Geometry check sheet. Reference: the model listing, model coordinates, mm. A direction names the side the tool comes from. Coordinates: 2 decimals unless noted, no trailing zeros. Loops run counter-clockwise (first coordinate to the right, second up) from the corner with the lowest first, then second, coordinate; pieces in that order, holes last. Notation, with made-up numbers: (-12.75, 11.25) -> (9.25, 11.25) arc R29 cw to (9.25, 31.25) -> close; hole circle Ø3 at (-25.5, -12.5). An arc over 180 degrees is marked (long way). Answer as a JSON object with one key per item and string values.
from build123d import *

# Parameters (mm, degrees)
SKETCH1_R           = 2.8
BOSS_EXTRUDE1_DEPTH = 1.5
SKETCH2_R           = 2.25
BOSS_EXTRUDE2_DEPTH = 7
SKETCH3_R           = 2.25
BOSS_EXTRUDE3_DEPTH = 15
CUT_EXTRUDE1_DEPTH  = 103.8
SKETCH5_R           = 1.8
CUT_EXTRUDE2_DEPTH  = 116.0000001
CUT_EXTRUDE3_DEPTH  = 13.8


with BuildPart() as part:
    # Sketch1 → Boss-Extrude1 (new body)
    with BuildSketch(Plane(origin=(0, 0, 0), x_dir=(1, 0, 0), z_dir=(0, 1, 0))):
        Circle(SKETCH1_R)
    extrude(amount=BOSS_EXTRUDE1_DEPTH)

    # Sketch2 → Boss-Extrude2 (add)
    with BuildSketch(Plane(origin=(0, 1.5, 0), x_dir=(1, 0, 0), z_dir=(0, 1, 0))):
        Circle(SKETCH2_R)
    extrude(amount=BOSS_EXTRUDE2_DEPTH)

    # Sketch3 → Boss-Extrude3 (add)
    with BuildSketch(Plane.XZ):
        Circle(SKETCH3_R)
    extrude(amount=BOSS_EXTRUDE3_DEPTH)

    # Sketch4 → Cut-Extrude1 (cut, through all)
    with BuildSketch(Plane(origin=(100, 0, 0), x_dir=(0, 0, -1), z_dir=(1, 0, 0))):
        with BuildLine():
            Line((0.5, -13.5), (0.5, -15))
            ThreePointArc((0.5, -15), (0, -15.5), (-0.5, -15))
            Line((-0.5, -15), (-0.5, -13.5))
            ThreePointArc((-0.5, -13.5), (0, -13), (0.5, -13.5))
        make_face()
        with BuildLine():
            Line((-0.5, 6.5), (-0.5, 8.5))
            ThreePointArc((-0.5, 8.5), (0, 9), (0.5, 8.5))
            Line((0.5, 8.5), (0.5, 6.5))
            ThreePointArc((0.5, 6.5), (0, 6), (-0.5, 6.5))
        make_face()
    extrude(amount=-CUT_EXTRUDE1_DEPTH, mode=Mode.SUBTRACT)

    # Sketch5 → Cut-Extrude2 (cut, through all)
    with BuildSketch(Plane(origin=(0, 100, 0), x_dir=(1, 0, 0), z_dir=(0, 1, 0))):
        Circle(SKETCH5_R)
    extrude(amount=-CUT_EXTRUDE2_DEPTH, mode=Mode.SUBTRACT)

    # Sketch6 → Cut-Extrude3 (cut, through all)
    with BuildSketch(Plane.XY.offset(10)):
        with BuildLine():
            Line((-0.5, -9), (-0.5, -6.191505656))
            ThreePointArc((-0.5, -6.191505656), (0, -5.691505656), (0.5, -6.191505656))
            Line((0.5, -6.191505656), (0.5, -9))
            ThreePointArc((0.5, -9), (0, -9.5), (-0.5, -9))
        make_face()
    extrude(amount=-CUT_EXTRUDE3_DEPTH, mode=Mode.SUBTRACT)


solid = part.part
1. Mould release check, pull along X, two halves, no side actions. Record for faces 4 (the face through (-2.8, 0.7, -0.1)), 5 (the face through (0, 8.5, 2)), 6 (the face through (1.717, -3.085, -0.541)): released by +X, released by -X, zero draft, split by the parting line, or undercut.
Evaluation:
{"face 4": "split by the parting line", "face 5": "zero draft", "face 6": "undercut"}
2. Tool access check on faces 1 (the face through (2.146, 4.951, -0.676)), 2 (the face through (2.146, -7.395, 0.676)), 3 (the face through (0, 8.5, -2)). Record the directions out of +Z, -Z, +X, -X, +Y, -Y that give a thin tool (end or side, any length) a straight path to the whole face; none if there is none.
Evaluation:
{"face 1": "+Y", "face 2": "-Y", "face 3": "+Z, -Z, +X, -X, +Y"}
3. Thickness scan on probe 1 along X at (y, z) = (-7.25, 0); probe 2 along Z at (x, y) = (0.5, -3.75). Record the ranges inside material, lowest first. Write a range as from..to.
Evaluation:
{"probe 1": "x = -2.25..-1.8, 1.8..2.25", "probe 2": "z = -2.19..-1.73, 1.73..2.19"}
4. Section check B-B, the plane z = 0. Record the boundary of the cut face in (x, y), then the cut area to 4 significant figures.
Evaluation:
{"outline": "(-2.8, 0) -> (-2.25, 0) -> (-2.25, -13) -> (-1.8, -13) -> (-1.8, 6) -> (-2.25, 6) -> (-2.25, 1.5) -> (-2.8, 1.5) -> close; (1.8, -13) -> (2.25, -13) -> (2.25, 0) -> (2.8, 0) -> (2.8, 1.5) -> (2.25, 1.5) -> (2.25, 6) -> (1.8, 6) -> close", "area": "18.75 mm^2"}
5. Depth check by flat-ended pin: P1, Ø1.5, axis at x = -1, z = -1, coming from the +Y side; P2, Ø3, axis at x = 0, z = 0, coming from the +Y side; P3, Ø0.5, axis at x = 2, y = 7.5, coming from the +Z side; P4, Ø0.5, axis at x = 2, y = -14.5, coming from the -Z side. Enter the tip coordinate at first touch or a pass-through.
Evaluation:
{"P1": "stops at y = 8.5", "P2": "passes through", "P3": "stops at z = 1.41", "P4": "stops at z = -1.41"}
6. Section check A-A, the plane x = 0. Record the boundary of the cut face in (y, z), then the cut area to 3 significant figures.
Evaluation:
{"outline": "(-15, -2.25) -> (-9.5, -2.25) -> (-9.5, -1.8) -> (-15, -1.8) -> close; (-15, 1.8) -> (-9.5, 1.8) -> (-9.5, 2.25) -> (-15, 2.25) -> close; (-5.69, -2.25) -> (0, -2.25) -> (0, -2.8) -> (1.5, -2.8) -> (1.5, -2.25) -> (8.5, -2.25) -> (8.5, -1.8) -> (-5.69, -1.8) -> close; (-5.69, 1.8) -> (8.5, 1.8) -> (8.5, 2.25) -> (1.5, 2.25) -> (1.5, 2.8) -> (0, 2.8) -> (0, 2.25) -> (-5.69, 2.25) -> close", "area": "19.4 mm^2"}
7. Section check D-D, the plane x = -1. Record the boundary of the cut face in (y, z), then the cut area to 3 significant figures.
Evaluation:
{"outline": "(-15, -2.02) -> (0, -2.02) -> (0, -2.62) -> (1.5, -2.62) -> (1.5, -2.02) -> (8.5, -2.02) -> (8.5, -1.5) -> (-15, -1.5) -> close; (-15, 1.5) -> (8.5, 1.5) -> (8.5, 2.02) -> (1.5, 2.02) -> (1.5, 2.62) -> (0, 2.62) -> (0, 2.02) -> (-15, 2.02) -> close", "area": "26.2 mm^2"}
8. Section check C-C, the plane y = -8. Record the boundary of the cut face in (x, z), then the cut area to 3 significant figures.
Evaluation:
{"outline": "(-0.5, -2.19) -> (-0.5, -1.73) arc R1.8 cw to (-0.5, 1.73) -> (-0.5, 2.19) arc R2.25 ccw to start; (0.5, -2.19) arc R2.25 ccw to (0.5, 2.19) -> (0.5, 1.73) arc R1.8 cw to (0.5, -1.73) -> close", "area": "4.82 mm^2"}
